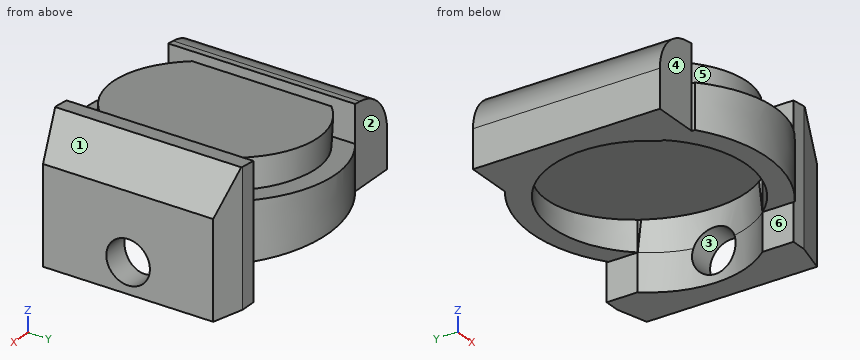
```python
from build123d import *
from OCP.BRepFilletAPI import BRepFilletAPI_MakeChamfer

# Parameters (mm, degrees)
SKETCH1_W                         = 3.81
SKETCH1_H                         = 15.24
BOSS_EXTRUDE1_DEPTH               = 8.128
BOSS_EXTRUDE1_2_DEPTH             = 8.128
CUT_EXTRUDE2_DEPTH                = 20.911072799
SKETCH12_R                        = 7.9375
MAGNET_DEPTH                      = 4.572
BOSS_EXTRUDE6_DEPTH               = 3.048
SKETCH14_R                        = 1.778
CUT_EXTRUDE4_DEPTH                = 2.54
CHAMFER3_SIZE                     = 2.54
CHAMFER3_SIZE2                    = 0.680590949
CHAMFER4_SIZE                     = 2.54
CHAMFER4_SIZE2                    = 0.680590949
CHAMFER5_SIZE                     = 3.302
CHAMFER5_SIZE2                    = 2.421231652
BOSS_EXTRUDE7_REACH               = 20.006
BOSS_EXTRUDE7_OFFSET_FROM_SURFACE = 3.048
FILLET1_R                         = 3.556


with BuildPart() as part:
    # Sketch1 → Boss-Extrude1 (new body)
    with BuildSketch(Plane.XY):
        with Locations((-8.001, 0)):
            Rectangle(SKETCH1_W, SKETCH1_H)
    extrude(amount=BOSS_EXTRUDE1_DEPTH)


with BuildPart() as body_2:
    # Sketch1 → Boss-Extrude1 2 (new body)
    with BuildSketch(Plane.XY):
        with Locations((8.001, 0)):
            Rectangle(SKETCH1_W, SKETCH1_H)
    extrude(amount=BOSS_EXTRUDE1_2_DEPTH)


with BuildPart() as cut_extrude2_tool:
    # Sketch6 → Cut-Extrude2 (new, through all)
    with BuildSketch(Plane(origin=(0, 7.62, 0), x_dir=(1, 0, 0), z_dir=(0, 1, 0))):
        Polygon((-9.906, -6.359826106), (9.906, -8.128), (-9.906, -8.128), align=None)
    extrude(amount=-CUT_EXTRUDE2_DEPTH)


with BuildPart() as part_1:
    add(part.part)

    # Cut-Extrude2: cut by cut_extrude2_tool
    add(cut_extrude2_tool.part, mode=Mode.SUBTRACT)

    # Cut-Loft1: read off the stored shape, not the designer's step
    # Cut-Loft1: loft between two sections, ruled curve by curve
    cut_loft1_from = [
        Edge.make_bspline([(-0.341139785, 7.934039191, 6.44843844), (15.401545931, 7.465303163, 7.853435709), (14.936513948, -8.402775219, 7.811932711), (-0.806171769, -7.934039191, 6.406935441), (-16.548857485, -7.465303163, 5.001938171), (-16.083825501, 8.402775219, 5.04344117), (-0.341139785, 7.934039191, 6.44843844)], [0, 0, 0, 0, 0.5, 0.5, 0.5, 1, 1, 1, 1], 3, [1, 0.333333333, 0.333333333, 1, 0.333333333, 0.333333333, 1]),
    ]
    cut_loft1_to = [
        Edge.make_bspline([(-0.164568393, 7.935793816, 0), (15.70701924, 8.264930602, 0), (16.036156025, -7.606657031, 0), (0.164568393, -7.935793816, 0), (-15.70701924, -8.264930602, 0), (-16.036156025, 7.606657031, 0), (-0.164568393, 7.935793816, 0)], [0, 0, 0, 0, 0.5, 0.5, 0.5, 1, 1, 1, 1], 3, [1, 0.333333333, 0.333333333, 1, 0.333333333, 0.333333333, 1]),
    ]
    cut_loft1 = Solid(Shell([*[Face.make_surface_from_curves(cut_loft1_from[k], cut_loft1_to[k]) for k in range(1)], Face(Wire(cut_loft1_from)), Face(Wire(cut_loft1_to))]))
    add(cut_loft1, mode=Mode.SUBTRACT)


with BuildPart() as body_2_1:
    add(body_2.part)

    # Cut-Extrude2: cut by cut_extrude2_tool
    add(cut_extrude2_tool.part, mode=Mode.SUBTRACT)

    # Cut-Loft1 2: loft between two sections, ruled curve by curve
    cut_loft1_2_from = [
        Edge.make_bspline([(-0.341139785, 7.934039191, 6.44843844), (15.401545931, 7.465303163, 7.853435709), (14.936513948, -8.402775219, 7.811932711), (-0.806171769, -7.934039191, 6.406935441), (-16.548857485, -7.465303163, 5.001938171), (-16.083825501, 8.402775219, 5.04344117), (-0.341139785, 7.934039191, 6.44843844)], [0, 0, 0, 0, 0.5, 0.5, 0.5, 1, 1, 1, 1], 3, [1, 0.333333333, 0.333333333, 1, 0.333333333, 0.333333333, 1]),
    ]
    cut_loft1_2_to = [
        Edge.make_bspline([(-0.164568393, 7.935793816, 0), (15.70701924, 8.264930602, 0), (16.036156025, -7.606657031, 0), (0.164568393, -7.935793816, 0), (-15.70701924, -8.264930602, 0), (-16.036156025, 7.606657031, 0), (-0.164568393, 7.935793816, 0)], [0, 0, 0, 0, 0.5, 0.5, 0.5, 1, 1, 1, 1], 3, [1, 0.333333333, 0.333333333, 1, 0.333333333, 0.333333333, 1]),
    ]
    cut_loft1_2 = Solid(Shell([*[Face.make_surface_from_curves(cut_loft1_2_from[k], cut_loft1_2_to[k]) for k in range(1)], Face(Wire(cut_loft1_2_from)), Face(Wire(cut_loft1_2_to))]))
    add(cut_loft1_2, mode=Mode.SUBTRACT)


with BuildPart() as body_3:
    # Sketch12 → Magnet (new body)
    with BuildSketch(Plane(origin=(-0.573655777, 0, 6.42768694), x_dir=(-0.9960410654107703, 0, -0.08889429686643446), z_dir=(0.08889429686643446, 0, -0.9960410654107703))):
        Circle(SKETCH12_R)
    extrude(amount=MAGNET_DEPTH)


with BuildPart() as body_4:
    # Sketch13 → Boss-Extrude6 (new body)
    with BuildSketch(Plane(origin=(0, 0, 0), x_dir=(-1, 0, 0), z_dir=(0, 0, -1))):
        with BuildLine():
            Line((-6.096, 5.08357062), (-6.096, 7.62))
            Line((-6.096, 7.62), (-9.906, 7.62))
            Line((-9.906, 7.62), (-9.906, -7.62))
            Line((-9.906, -7.62), (-6.096, -7.62))
            Line((-6.096, -7.62), (-6.096, -5.08357062))
            ThreePointArc((-6.096, -5.08357062), (-7.9375, 0), (-6.096, 5.08357062))
        make_face()
    extrude(amount=BOSS_EXTRUDE6_DEPTH)


with BuildPart() as cut_extrude4_tool:
    # Sketch14 → Cut-Extrude4 (new body)
    with BuildSketch(Plane(origin=(9.906, 0, 0), x_dir=(0, 0, -1), z_dir=(1, 0, 0))):
        with Locations((0.597062067, -1.1e-08)):
            Circle(SKETCH14_R)
    extrude(amount=-CUT_EXTRUDE4_DEPTH)


with BuildPart() as body_2_2:
    add(body_2_1.part)

    # Cut-Extrude4: cut by cut_extrude4_tool
    add(cut_extrude4_tool.part, mode=Mode.SUBTRACT)

    # Chamfer3: one chamfer whose edges measure the first distance from different faces: ONE call of the kernel's chamfer builder (chamfer() names one face for all edges)
    chamfer3_edges_1 = [body_2_2.edges().sort_by_distance(p)[0] for p in [
        (9.906, -7.62, 4.064),
    ]]
    chamfer3_side_1 = [body_2_2.faces().sort_by_distance(p)[0] for p in [
        (8.014566329, -7.62, 3.979597021),
    ]]
    chamfer3_edges_2 = [body_2_2.edges().sort_by_distance(p)[0] for p in [
        (9.906, 7.62, 4.064),
    ]]
    chamfer3_side_2 = [body_2_2.faces().sort_by_distance(p)[0] for p in [
        (8.014566329, 7.62, 3.979597021),
    ]]
    chamfer3 = BRepFilletAPI_MakeChamfer(body_2_2.part.solid().wrapped)
    for e in chamfer3_edges_1:
        chamfer3.Add(CHAMFER3_SIZE, CHAMFER3_SIZE2, e.wrapped, chamfer3_side_1[0].wrapped)  # the first distance lies on this face
    for e in chamfer3_edges_2:
        chamfer3.Add(CHAMFER3_SIZE, CHAMFER3_SIZE2, e.wrapped, chamfer3_side_2[0].wrapped)  # the first distance lies on this face
    add(Compound.cast(chamfer3.Shape()), mode=Mode.REPLACE)

    # Chamfer5
    chamfer5_edges = [body_2_2.edges().sort_by_distance(p)[0] for p in [
        (9.906, 0, 8.128),
    ]]
    chamfer5_side = [body_2_2.faces().sort_by_distance(p)[0] for p in [
        (9.906, 0, 4.157766254),
    ]]
    chamfer(chamfer5_edges, length=CHAMFER5_SIZE, length2=CHAMFER5_SIZE2, reference=chamfer5_side[0])

    # Boss-Extrude7: up to this face of the body (flat: up to its plane, moved by the offset)
    boss_extrude7_end = Plane(body_2_2.part.faces().sort_by_distance((6.795040928, 0, 7.8503543))[0]).offset(-BOSS_EXTRUDE7_OFFSET_FROM_SURFACE)
    # Sketch15 → Boss-Extrude7 (add, up to the picked face)
    with BuildSketch(Plane.XY, mode=Mode.PRIVATE) as boss_extrude7_sk1:
        with BuildLine():
            Line((6.096, 5.08357062), (6.096, 7.471449808))
            add(Edge.make_bspline(
                [(6.096, 7.471449808), (5.930756217, 7.591123534), (5.255615528, 8.051037173), (3.293003266, 9.079390192), (1.283010021, 9.48240548), (-0.107834445, 9.483073279), (-1.498678912, 9.483741079), (-3.43762918, 9.094971238), (-5.325260948, 8.130204629), (-5.94396227, 7.728072028), (-6.096, 7.623571521)],
                knots=[0.900690867, 0.900690867, 0.900690867, 0.900690867, 0.909893147, 0.9375, 1, 1, 1, 1.0625, 1.087339124, 1.095618826, 1.095618826, 1.095618826, 1.095618826], degree=3))
            Line((-6.096, 7.623571521), (-6.096001081, 5.083571521))
            add(Edge.make_bspline(
                [(6.096, 5.08357062), (5.93161291, 5.274891544), (5.758408134, 5.458513784), (5.199745975, 5.997244915), (4.788453523, 6.323024277), (4.121406265, 6.751856672), (3.889862409, 6.885002693), (3.419802681, 7.125246454), (3.180186729, 7.23314886), (2.447832586, 7.520869047), (1.940077624, 7.665345536), (0.893913787, 7.852965093), (0.366394093, 7.894488776), (-0.165582558, 7.883517088), (-0.697559209, 7.8725454), (-1.219532269, 7.809382621), (-1.988103649, 7.639571774), (-2.241878196, 7.570363771), (-2.744485351, 7.406164502), (-2.993938175, 7.310744438), (-3.718584086, 6.991700252), (-4.175623921, 6.734186385), (-5.038069326, 6.130349805), (-5.444832888, 5.781030811), (-5.906820855, 5.29786321), (-6.002858614, 5.191954979), (-6.096001081, 5.083571521)],
                knots=[0.860122022, 0.860122022, 0.860122022, 0.860122022, 0.875, 0.875, 0.90625, 0.90625, 0.921875, 0.921875, 0.9375, 0.9375, 0.96875, 0.96875, 1, 1, 1, 1.03125, 1.03125, 1.046875, 1.046875, 1.0625, 1.0625, 1.09375, 1.09375, 1.125, 1.125, 1.133513625, 1.133513625, 1.133513625, 1.133513625], degree=3))
        make_face()
    boss_extrude7_tool1 = split(extrude(boss_extrude7_sk1.sketch, amount=BOSS_EXTRUDE7_REACH, mode=Mode.PRIVATE), bisect_by=boss_extrude7_end, keep=Keep.BOTH, mode=Mode.PRIVATE)
    # Sketch15 → Boss-Extrude7 (add, up to the picked face)
    with BuildSketch(Plane.XY, mode=Mode.PRIVATE) as boss_extrude7_sk2:
        with BuildLine():
            add(Edge.make_bspline(
                [(-6.096, -5.334665385), (-6.001608062, -5.440026559), (-5.904161756, -5.543205008), (-5.428535567, -6.020913198), (-5.021324344, -6.355746552), (-4.367831042, -6.794427859), (-4.142640685, -6.930176212), (-3.677224948, -7.180264747), (-3.435889004, -7.294952261), (-2.704038324, -7.599333248), (-2.202060233, -7.75220516), (-1.170288992, -7.959061026), (-0.636413301, -8.012110875), (0.415017809, -8.012485804), (0.937476738, -7.961532915), (1.716181401, -7.806841712), (1.975144289, -7.741886149), (2.479947756, -7.588440875), (2.974576658, -7.410991551), (3.449201256, -7.186347645), (3.913706318, -6.937829508), (4.141960005, -6.800903506), (4.803088275, -6.358194944), (5.208510395, -6.024190383), (5.760001551, -5.471897601), (5.932187446, -5.282339739), (6.096, -5.08357062)],
                knots=[1.366624359, 1.366624359, 1.366624359, 1.366624359, 1.375, 1.375, 1.40625, 1.40625, 1.421875, 1.421875, 1.4375, 1.4375, 1.46875, 1.46875, 1.5, 1.5, 1.53125, 1.53125, 1.546875, 1.546875, 1.5625, 1.578125, 1.578125, 1.59375, 1.59375, 1.625, 1.625, 1.640183323, 1.640183323, 1.640183323, 1.640183323], degree=3))
            Line((6.096, -5.08357062), (6.096, -7.72253105))
            add(Edge.make_bspline(
                [(-6.096, -7.874665385), (-5.811745982, -8.069955065), (-5.191368312, -8.452655749), (-3.271071363, -9.379610796), (-0.11139785, -10.010823197), (3.138794467, -9.363488053), (5.12304575, -8.377449625), (5.814796936, -7.926184012), (6.096, -7.72253105)],
                knots=[1.404521499, 1.404521499, 1.404521499, 1.404521499, 1.420146511, 1.4375, 1.5, 1.5625, 1.583974967, 1.599599961, 1.599599961, 1.599599961, 1.599599961], degree=3))
            Line((-6.096, -7.874665385), (-6.096, -5.334665385))
        make_face()
    boss_extrude7_tool2 = split(extrude(boss_extrude7_sk2.sketch, amount=BOSS_EXTRUDE7_REACH, mode=Mode.PRIVATE), bisect_by=boss_extrude7_end, keep=Keep.BOTH, mode=Mode.PRIVATE)

    add(part_1.part)  # Boss-Extrude7 merges part

    add(body_3.part)  # Boss-Extrude7 merges body 3


with BuildPart() as body_4_1:
    add(body_4.part)

    # Cut-Extrude4: cut by cut_extrude4_tool
    add(cut_extrude4_tool.part, mode=Mode.SUBTRACT)

    # Chamfer4: one chamfer whose edges measure the first distance from different faces: ONE call of the kernel's chamfer builder (chamfer() names one face for all edges)
    chamfer4_edges_1 = [body_4_1.edges().sort_by_distance(p)[0] for p in [
        (9.906, -7.62, -1.524),
    ]]
    chamfer4_side_1 = [body_4_1.faces().sort_by_distance(p)[0] for p in [
        (8.001, -7.62, -1.524),
    ]]
    chamfer4_edges_2 = [body_4_1.edges().sort_by_distance(p)[0] for p in [
        (9.906, 7.62, -1.524),
    ]]
    chamfer4_side_2 = [body_4_1.faces().sort_by_distance(p)[0] for p in [
        (8.001, 7.62, -1.524),
    ]]
    chamfer4 = BRepFilletAPI_MakeChamfer(body_4_1.part.solid().wrapped)
    for e in chamfer4_edges_1:
        chamfer4.Add(CHAMFER4_SIZE, CHAMFER4_SIZE2, e.wrapped, chamfer4_side_1[0].wrapped)  # the first distance lies on this face
    for e in chamfer4_edges_2:
        chamfer4.Add(CHAMFER4_SIZE, CHAMFER4_SIZE2, e.wrapped, chamfer4_side_2[0].wrapped)  # the first distance lies on this face
    add(Compound.cast(chamfer4.Shape()), mode=Mode.REPLACE)


with BuildPart() as body_2_3:
    add(body_2_2.part)

    add(body_4_1.part)  # Boss-Extrude7 merges body 4
    add(boss_extrude7_tool1.solids().sort_by(Axis((5.966385, 6.27751, 0), (0, 0, 1)))[0])
    add(boss_extrude7_tool2.solids().sort_by(Axis((0.034935, -8.049766, 0), (0, 0, 1)))[0])

    # Fillet1
    fillet1_edges = [body_2_3.edges().sort_by_distance(p)[0] for p in [
        (-9.906, 0, 6.359826106),
    ]]
    fillet(fillet1_edges, radius=FILLET1_R)


solid = body_2_3.part
```
CAD build for the part. Positions are in the model's coordinates, mm. Face numbers are marked on the shaded views. A direction names the side the tool comes from. Round coordinates to 2 decimals unless told otherwise and drop trailing zeros. Write each loop counter-clockwise with the first axis right and the second up, starting at its lowest first coordinate (ties: lowest second). Pieces come first, ordered by that corner, then holes. Notation, with made-up numbers: (66, 29.25) - (100, 29.25) arc R23 ccw to (100, 54.25) - close; hole circle Ø8 at (25, 80). An arc over 180 degrees is marked (long way). Return JSON: item names as keys, results as strings. Group by question number.
Item 1: Flat gauge pins, fed straight in: pin 1 Ø0.6 at (x, z) = (7, 1) entering from +Y; pin 2 Ø1.3 at (y, z) = (-5.5, -1) entering from -X; pin 3 Ø2 at (x, z) = (-1, 6.5) entering from +Y. Where does each tip first touch, or does it go through?
Item 2: 3-axis set-ups, long thin cutter, end or side, ignore diameter. For the marked faces 4, 5 and 6: which of +Z, -Z, +X, -X, +Y, -Y reach the whole face in a straight line?
Item 3: Mould opens along Z. For the marked faces 1, 2 and 3 say: +Z half, -Z half, draft (parallel to the pull), parting line (faces both ways), or undercut.
Item 4: Band-saw the part on A-A on z = -2. List the corners of the cut face in (x, y) (1 decimal), plus the area to 3 significant figures.
Item 5: Band-saw the part on C-C on x = 8.75. List the corners of the cut face in (y, z), plus the area to 3 significant figures.
Item 6: Band-saw the part on B-B on x = 5.5. State how many separate pieces and enclosed holes the cut face has, plus the area to 3 significant figures.
Item 7: Probe probe 1 along Y at (x, z) = (0.75, 1.25); probe 2 along X at (y, z) = (-1.25, 0.75); probe 3 along Z at (x, y) = (8.3, 0). List the from-to ranges inside material, lowest first.
Resolved:
{
 "1": {"pin 1": "stops at y = 7.62", "pin 2": "stops at x = 6.1", "pin 3": "stops at y = 7.94"},
 "2": {"face 4": "+Z, -Z, -X, -Y", "face 5": "none", "face 6": "-Z, -X, +Y, -Y"},
 "3": {"face 1": "+Z half", "face 2": "draft", "face 3": "undercut"},
 "4": {"outline": "(6.1, -7.6) - (7.4, -7.6) - (9.9, -6.9) - (9.9, -1.1) - (7.9, -1.1) arc R7.9 cw to (6.1, -5.1) - close; (6.1, 5.1) arc R7.9 cw to (7.9, 1.1) - (9.9, 1.1) - (9.9, 6.9) - (7.4, 7.6) - (6.1, 7.6) - close", "area": "39.2 mm²"},
 "5": {"outline": "(-7.25, -3.05) - (7.25, -3.05) - (7.25, 6.31) - (-7.25, 6.31) - close; hole circle Ø3.56 at (0, -0.6)", "area": "126 mm²"},
 "6": {"separate pieces": "3", "enclosed holes": "0", "area": "70.1 mm²"},
 "7": {"probe 1": "y = -9.7 to -7.97, 7.85 to 9.45", "probe 2": "x = -9.91 to -7.9, 7.77 to 9.91", "probe 3": "z = -3.05 to -2.38, 1.18 to 6.88"}
}
